Verification items for the finished model (mm, model axes). Give positions to 0.01 mm unless a question says otherwise; leave off trailing zeros. Write each loop counter-clockwise with the first axis right and the second up, starting at its lowest first coordinate (ties: lowest second). Pieces come first, ordered by that corner, then holes. Notation, with made-up numbers: (-13.75, -2.75) -> (8.25, -2.75) arc R25 cw to (8.25, 17.25) -> close; hole circle Ø8 at (25.5, -20.75). An arc over 180 degrees is marked (long way). Use CSV: the item, a comma, the result in double quotes. Start each with the question number.
Autodesk Inventor part; units mm, degrees
ref_plane "YZ Plane" through (0, 0, 0) normal (1, 0, 0) x (0, 1, 0)
ref_plane "XZ Plane" through (0, 0, 0) normal (0, 1, 0) x (-1, 0, 0)
ref_plane "XY Plane" through (0, 0, 0) normal (0, 0, 1) x (1, 0, 0)
sketch "Sketch1" plane through (0, 0, 0) normal (0, 0, 1) x (1, 0, 0)
  line L0 (0, 0) -> (25.4, 0)
  line L1 (25.4, 0) -> (25.4, 25.4)
  line L2 (25.4, 25.4) -> (0, 25.4)
  line L3 (0, 25.4) -> (0, 0)
  dimension "d0" = 25.4
  dimension "d1" = 25.4
extrude "Extrusion1" add sketch "Sketch1" along normal blind 838.2
sketch "Sketch2" plane through (25.4, 0, 0) normal (1, 0, 0) x (0, 0, -1)
  line L0 (-838.2, 0) -> (-838.2, 25.4)
  circle A0 centre (-800.1, 12.7) radius 7.9375
  circle A1 centre (-823.9125, 12.7) radius 2.3813
  circle A2 centre (-776.2875, 12.7) radius 2.3812
  dimension "d4" = 15.875
  dimension "d5" = 38.1
  dimension "d8" = 4.7625
  dimension "d9" = 4.7625
  dimension "d10" = 23.8125
  dimension "d11" = 23.8125
extrude "Extrusion3" cut sketch "Sketch2" against normal blind 25.4
equation "\"d11\" = d10"
properties part number "utilityarm1x1"
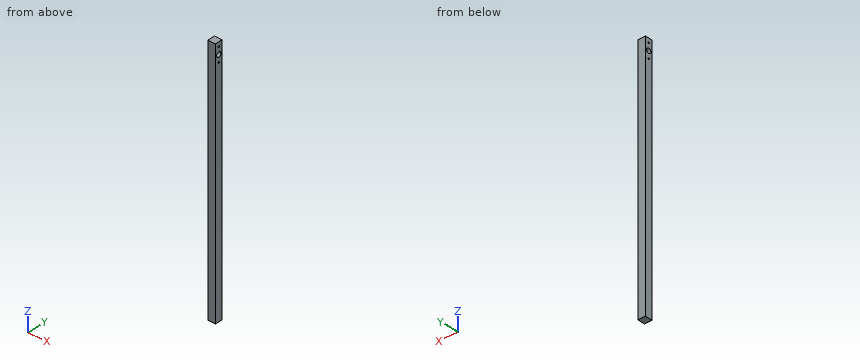
(1) Go/stop test with a flat-tipped pin: pin 1 (4 mm diameter, centred on y = 12.7, z = 823.91, fed in from -X). Record where the tip stops, or that it passes through.
(2) Section check A-A on z = 800.1. Record the cut outline in (x, y).
(3) Thickness scan on line 1 (Y direction, x = 16, z = 800.1); line 2 (Z direction, x = 10.25, y = 15.25); line 3 (Z direction, x = 10.5, y = 19). Record the ranges inside material, lowest first. Write a range as from..to.
Data:
1,pin 1,"passes through"
2,outline,"(0, 0) -> (25.4, 0) -> (25.4, 4.76) -> (0, 4.76) -> close; (0, 20.64) -> (25.4, 20.64) -> (25.4, 25.4) -> (0, 25.4) -> close"
3,line 1,"y = 0..4.76, 20.64..25.4"
3,line 2,"z = 0..792.58, 807.62..838.2"
3,line 3,"z = 0..795.27, 804.93..838.2"
